```python
from build123d import *

# Parameters (mm, degrees)
SKETCH1_W           = 50
SKETCH1_H           = 20
BOSS_EXTRUDE1_DEPTH = 33
SKETCH2_R           = 2.65
CUT_EXTRUDE1_DEPTH  = 64.158530699
BOSS_EXTRUDE2_DEPTH = 25
CUT_EXTRUDE8_DEPTH  = 80.14543575
SKETCH10_R          = 11.5
CUT_EXTRUDE10_DEPTH = 78.5112895
FILLET1_R           = 1
SKETCH3_R           = 5.1
SKETCH3_R_2         = 1.85
CUT_EXTRUDE11_DEPTH = 80.14543575
SKETCH11_R          = 11.15
CUT_EXTRUDE12_DEPTH = 3.8
CUT_EXTRUDE14_DEPTH = 5


with BuildPart() as part:
    # Sketch1 → Boss-Extrude1 (new body)
    with BuildSketch(Plane(origin=(0, 0, 0), x_dir=(1, 0, 0), z_dir=(0, 1, 0))):
        with Locations((25, 10)):
            Rectangle(SKETCH1_W, SKETCH1_H)
    extrude(amount=BOSS_EXTRUDE1_DEPTH)

    # Sketch2 → Cut-Extrude1 (cut, through all)
    with BuildSketch(Plane.XY):
        with Locations((6, 20)):
            Circle(SKETCH2_R)
        with Locations((44, 20)):
            Circle(SKETCH2_R)
    extrude(amount=-CUT_EXTRUDE1_DEPTH, mode=Mode.SUBTRACT)

    # Sketch7 → Boss-Extrude2 (add)
    with BuildSketch(Plane(origin=(0, 33, 0), x_dir=(1, 0, 0), z_dir=(0, 1, 0))):
        Polygon((50, 0), (50, 20), (0, 20), (0, 0), (6, 0), (6, 12), (44, 12), (44, 0), align=None)
    extrude(amount=BOSS_EXTRUDE2_DEPTH)

    # Sketch8 → Cut-Extrude8 (cut, through all)
    with BuildSketch(Plane.ZY):
        Polygon((0, 58), (0, 33), (-12, 58), align=None)
    extrude(amount=-CUT_EXTRUDE8_DEPTH, mode=Mode.SUBTRACT)

    # Sketch10 → Cut-Extrude10 (cut, through all)
    with BuildSketch(Plane.XY.offset(-12)):
        with Locations((25, 40)):
            Circle(SKETCH10_R)
    extrude(amount=CUT_EXTRUDE10_DEPTH, mode=Mode.SUBTRACT)

    # Fillet1
    fillet1_edges = [part.edges().sort_by_distance(p)[0] for p in [
        (6, 33, -6),
        (10.937928102, 33, -12),
        (6, 45.5, -12),
        (44, 33, -6),
        (44, 45.5, -12),
        (0, 58, -16),
        (50, 58, -16),
        (39.062071898, 33, -12),
        (25, 28.5, -12),
    ]]
    fillet(fillet1_edges, radius=FILLET1_R)

    # Sketch3 → Cut-Extrude11 (cut, through all)
    with BuildSketch(Plane.XY):
        with Locations((25, 20)):
            Circle(SKETCH3_R)
        with Locations((19.413856429, 25.586143571)):
            Circle(SKETCH3_R_2)
        with Locations((30.586143571, 25.586143571)):
            Circle(SKETCH3_R_2)
        with Locations(Location((30.586143571, 14.413856429, 0), (0, 0, 180))):
            Circle(SKETCH3_R_2)
        with Locations(Location((19.413856429, 14.413856429, 0), (0, 0, 180))):
            Circle(SKETCH3_R_2)
    extrude(amount=-CUT_EXTRUDE11_DEPTH, mode=Mode.SUBTRACT)

    # Sketch11 → Cut-Extrude12 (cut)
    with BuildSketch(Plane(origin=(0, 0, -20), x_dir=(-1, 0, 0), z_dir=(0, 0, -1))):
        with Locations((-25, 20)):
            Circle(SKETCH11_R)
    extrude(amount=-CUT_EXTRUDE12_DEPTH, mode=Mode.SUBTRACT)

    # Sketch12 → Cut-Extrude14 (cut)
    # profile 1 of 16: a face of its own
    with BuildSketch(Plane.XY):
        with BuildLine():
            ThreePointArc((21.888730163, 28.061017306), (16.938982694, 28.061017306), (16.938982694, 23.111269837))
            Line((16.938982694, 23.111269837), (19.413856429, 25.586143571))
            Line((19.413856429, 25.586143571), (21.888730163, 28.061017306))
        make_face()
    # profile 2 of 16: a face of its own
    with BuildSketch(Plane.XY):
        with BuildLine():
            Line((21.888730163, 28.061017306), (19.413856429, 25.586143571))
            Line((19.413856429, 25.586143571), (21.393755416, 23.606244584))
            ThreePointArc((21.393755416, 23.606244584), (22.039987111, 24.153110124), (22.76777875, 24.585541221))
            ThreePointArc((22.76777875, 24.585541221), (22.877144471, 25.080539044), (22.913856429, 25.586143571))
            ThreePointArc((22.913856429, 25.586143571), (22.647434792, 26.925535585), (21.888730163, 28.061017306))
        make_face()
    # profile 3 of 16: a face of its own
    with BuildSketch(Plane.XY):
        with BuildLine():
            Line((24.851898324, 25.097849144), (21.888730163, 28.061017306))
            ThreePointArc((21.888730163, 28.061017306), (22.647434792, 26.925535585), (22.913856429, 25.586143571))
            ThreePointArc((22.913856429, 25.586143571), (22.877144471, 25.080539044), (22.76777875, 24.585541221))
            ThreePointArc((22.76777875, 24.585541221), (23.78258505, 24.952565077), (24.851898324, 25.097849144))
        make_face()
    # profile 4 of 16: a face of its own
    with BuildSketch(Plane.XY):
        with BuildLine():
            Line((19.413856429, 25.586143571), (16.938982694, 23.111269837))
            ThreePointArc((16.938982694, 23.111269837), (18.555631148, 22.192996158), (20.414458779, 22.23222125))
            ThreePointArc((20.414458779, 22.23222125), (20.846889876, 22.960012889), (21.393755416, 23.606244584))
            Line((21.393755416, 23.606244584), (19.413856429, 25.586143571))
        make_face()
    # profile 5 of 16: a face of its own
    with BuildSketch(Plane.XY):
        with BuildLine():
            Line((16.938982694, 23.111269837), (19.902150856, 20.148101676))
            ThreePointArc((19.902150856, 20.148101676), (20.047434923, 21.21741495), (20.414458779, 22.23222125))
            ThreePointArc((20.414458779, 22.23222125), (18.555631148, 22.192996158), (16.938982694, 23.111269837))
        make_face()
    # profile 6 of 16: a face of its own
    with BuildSketch(Plane.XY):
        with BuildLine():
            ThreePointArc((25.148101676, 25.097849144), (26.21741495, 24.952565077), (27.23222125, 24.585541221))
            ThreePointArc((27.23222125, 24.585541221), (27.192996158, 26.444368852), (28.111269837, 28.061017306))
            Line((28.111269837, 28.061017306), (25.148101676, 25.097849144))
        make_face()
    # profile 7 of 16: a face of its own
    with BuildSketch(Plane.XY):
        with BuildLine():
            ThreePointArc((27.23222125, 24.585541221), (27.960012889, 24.153110124), (28.606244584, 23.606244584))
            Line((28.606244584, 23.606244584), (30.586143571, 25.586143571))
            Line((30.586143571, 25.586143571), (28.111269837, 28.061017306))
            ThreePointArc((28.111269837, 28.061017306), (27.192996158, 26.444368852), (27.23222125, 24.585541221))
        make_face()
    # profile 8 of 16: a face of its own
    with BuildSketch(Plane.XY):
        with BuildLine():
            Line((28.111269837, 28.061017306), (30.586143571, 25.586143571))
            Line((30.586143571, 25.586143571), (33.061017306, 23.111269837))
            ThreePointArc((33.061017306, 23.111269837), (33.819721935, 24.246751558), (34.086143571, 25.586143571))
            ThreePointArc((34.086143571, 25.586143571), (31.925535585, 28.819721935), (28.111269837, 28.061017306))
        make_face()
    # profile 9 of 16: a face of its own
    with BuildSketch(Plane.XY):
        with BuildLine():
            Line((30.586143571, 25.586143571), (28.606244584, 23.606244584))
            ThreePointArc((28.606244584, 23.606244584), (29.153110124, 22.960012889), (29.585541221, 22.23222125))
            ThreePointArc((29.585541221, 22.23222125), (31.444368852, 22.192996158), (33.061017306, 23.111269837))
            Line((33.061017306, 23.111269837), (30.586143571, 25.586143571))
        make_face()
    # profile 10 of 16: a face of its own
    with BuildSketch(Plane.XY):
        with BuildLine():
            ThreePointArc((33.061017306, 23.111269837), (31.444368852, 22.192996158), (29.585541221, 22.23222125))
            ThreePointArc((29.585541221, 22.23222125), (29.952565077, 21.21741495), (30.097849144, 20.148101676))
            Line((30.097849144, 20.148101676), (33.061017306, 23.111269837))
        make_face()
    # profile 11 of 16: a face of its own
    with BuildSketch(Plane.XY):
        with BuildLine():
            ThreePointArc((27.23222125, 15.414458779), (27.192996158, 13.555631148), (28.111269837, 11.938982694))
            ThreePointArc((28.111269837, 11.938982694), (31.925535585, 11.180278065), (34.086143571, 14.413856429))
            ThreePointArc((34.086143571, 14.413856429), (33.819721928, 15.753248458), (33.061017281, 16.888730188))
            ThreePointArc((33.061017281, 16.888730188), (31.444368835, 17.807003846), (29.585541221, 17.76777875))
            ThreePointArc((29.585541221, 17.76777875), (29.153110124, 17.039987111), (28.606244584, 16.393755416))
            ThreePointArc((28.606244584, 16.393755416), (27.960012889, 15.846889876), (27.23222125, 15.414458779))
        make_face()
        with BuildLine():
            ThreePointArc((32.436143571, 14.413856429), (29.878179221, 12.704679293), (29.277996026, 15.722003974))
            ThreePointArc((29.277996026, 15.722003974), (31.294107921, 16.123033564), (32.436143571, 14.413856429))
        make_face(mode=Mode.SUBTRACT)
    # profile 12 of 16: a face of its own
    with BuildSketch(Plane.XY):
        with BuildLine():
            ThreePointArc((27.23222125, 15.414458779), (26.21741495, 15.047434923), (25.148101676, 14.902150856))
            Line((25.148101676, 14.902150856), (28.111269837, 11.938982694))
            ThreePointArc((28.111269837, 11.938982694), (27.192996158, 13.555631148), (27.23222125, 15.414458779))
        make_face()
    # profile 13 of 16: a face of its own
    with BuildSketch(Plane.XY):
        with BuildLine():
            ThreePointArc((22.76777875, 15.414458779), (22.039987111, 15.846889876), (21.393755416, 16.393755416))
            ThreePointArc((21.393755416, 16.393755416), (20.846889876, 17.039987111), (20.414458779, 17.76777875))
            ThreePointArc((20.414458779, 17.76777875), (18.555631148, 17.807003842), (16.938982694, 16.888730163))
            ThreePointArc((16.938982694, 16.888730163), (16.9389827, 11.938982689), (21.888730174, 11.938982705))
            ThreePointArc((21.888730174, 11.938982705), (22.647434795, 13.074464422), (22.913856429, 14.413856429))
            ThreePointArc((22.913856429, 14.413856429), (22.877144471, 14.919460956), (22.76777875, 15.414458779))
        make_face()
        with BuildLine():
            ThreePointArc((21.263856429, 14.413856429), (17.704679293, 13.705892079), (20.722003974, 15.722003974))
            ThreePointArc((20.722003974, 15.722003974), (21.123033564, 15.121820779), (21.263856429, 14.413856429))
        make_face(mode=Mode.SUBTRACT)
    # profile 14 of 16: a face of its own
    with BuildSketch(Plane.XY):
        with BuildLine():
            ThreePointArc((24.851898324, 14.902150856), (23.78258505, 15.047434923), (22.76777875, 15.414458779))
            ThreePointArc((22.76777875, 15.414458779), (22.877144471, 14.919460956), (22.913856429, 14.413856429))
            ThreePointArc((22.913856429, 14.413856429), (22.647434795, 13.074464422), (21.888730174, 11.938982705))
            Line((21.888730174, 11.938982705), (24.851898324, 14.902150856))
        make_face()
    # profile 15 of 16: a face of its own
    with BuildSketch(Plane.XY):
        with BuildLine():
            ThreePointArc((16.938982694, 16.888730163), (18.555631148, 17.807003842), (20.414458779, 17.76777875))
            ThreePointArc((20.414458779, 17.76777875), (20.047434923, 18.78258505), (19.902150856, 19.851898324))
            Line((19.902150856, 19.851898324), (16.938982694, 16.888730163))
        make_face()
    # profile 16 of 16: a face of its own
    with BuildSketch(Plane.XY):
        with BuildLine():
            Line((33.061017281, 16.888730188), (30.097849144, 19.851898324))
            ThreePointArc((30.097849144, 19.851898324), (29.952565077, 18.78258505), (29.585541221, 17.76777875))
            ThreePointArc((29.585541221, 17.76777875), (31.444368835, 17.807003846), (33.061017281, 16.888730188))
        make_face()
    extrude(amount=-CUT_EXTRUDE14_DEPTH, mode=Mode.SUBTRACT)


solid = part.part
```
Geometry: final body of the model. Coordinates: model frame, mm. A direction names the side the tool comes from. Give positions to 0.01 mm unless a question says otherwise; leave off trailing zeros. Order: outer loops, then holes, each group sorted by start corner. A loop starts at its lowest first (then second) coordinate and runs counter-clockwise, first axis right, second up. Notation, with made-up numbers: M 34,-29 L 56,-29 A22 ccw 56,-9 Z; hole C 70,-12.5 d11. An arc over 180 degrees is marked long. Answer as CSV lines item,"result". Start each with the question number.
1) Cut plane C-C (z = -2.5). State how many separate pieces and enclosed holes the cut face has, then the cut area to 3 significant figures.
2) Cut plane D-D (y = 40.5). Output: boundary loops of the cut face in (x, z).
3) Set-up query: faces 4 (the flat face through (26.61, 13.44, -2.46)), 5 (the flat face through (25, 44, -12)), 6 (the flat face through (0, 28, -10)). Return all of +Z, -Z, +X, -X, +Y, -Y with unobstructed straight access to the full face (end or side cutting, diameter ignored); none if empty.
4) Line query: line 1 (X direction, y = 14.5, z = -15.75); line 2 (X direction, y = 45, z = -10); line 3 (X direction, y = 14.5, z = -1.5). Output: solid intervals per line, ascending. Write a range as from..to.
5) Cut plane B-B (y = 53). Output: boundary loops of the cut face in (x, z).
6) First-contact query: P1, Ø3, axis at x = 12, z = -8, coming from the +Y side; P2, Ø8.5, axis at x = 26, y = 39.5, coming from the +Z side. Flat tips, straight axial feed; report the tip coordinate or a pass-through.
7) Cut plane A-A (z = -7). Output: boundary loops of the cut face in (x, y).
8) Mould query, pull axis Y, two halves, no side actions, for faces 1 (the flat face through (50, 28, -10)), 2 (the flat face through (47.229, 45.325, -5.916)), 3 (the cylindrical face through (17.705, 15.122, -10.522)). Classes: +Y half, -Y half, draft (parallel to the pull), parting line (faces both ways), or undercut.
Findings below:
1,separate pieces,"1"
1,enclosed holes,"3"
1,area,"1,360 mm²"
2,outline,"M 0,-20 L 50,-20 L 50,-3.6 L 44,-3.6 L 44,-11 A1 cw 43,-12 L 7,-12 A1 cw 6,-11 L 6,-3.6 L 0,-3.6 Z"
3,face 4,"+Z"
3,face 5,"+Z, +Y"
3,face 6,"+Z, -Z, -X, +Y, -Y"
4,line 1,"x = 0..17.57, 21.26..28.74, 32.43..50"
4,line 2,"x = 0..6, 44..50"
4,line 3,"x = 0..15.91, 24.45..25.55, 34.09..50"
5,outline,"M 0,-20 L 50,-20 L 50,-9.6 L 44,-9.6 L 44,-11 A1 cw 43,-12 L 7,-12 A1 cw 6,-11 L 6,-9.6 L 0,-9.6 Z"
6,P1,"stops at y = 33"
6,P2,"stops at z = -12"
7,outline,"M 0,0 L 50,0 L 50,47.58 L 44,47.58 L 44,34 A1 cw 43,33 L 34.12,33 A11.5 cw 15.88,33 L 7,33 A1 cw 6,34 L 6,47.58 L 0,47.58 Z; hole C 6,20 d5.3; hole C 19.41,14.41 d3.7; hole C 19.41,25.59 d3.7; hole C 25,20 d10.2; hole C 30.59,14.41 d3.7; hole C 30.59,25.59 d3.7; hole C 44,20 d5.3"
8,face 1,"draft"
8,face 2,"+Y half"
8,face 3,"undercut"
